Read the model definition and answer for the solid it produces. Units are mm, in the model's axes. A direction names the side the tool comes from. Coordinates: 2 decimals unless noted, no trailing zeros. Order: outer loops, then holes, each group sorted by start corner. A loop starts at its lowest first (then second) coordinate and runs counter-clockwise, first axis right, second up. Notation, with made-up numbers: M 2.5,-35.75 L 54.5,-35.75 A19 cw 54.5,-13.75 Z; hole C -34,49 d7. An arc over 180 degrees is marked long. Use a Markdown table: item, result. Add a question column.
1) Find section C-C on z = 15. Write down the section's boundary in (x, y).
2) The mould has two halves that part along X. Classify faces 1 (the face through (-9, 15, 19)), 2 (the face through (-20, 10, 0)), 3 (the face through (0, 10, -20)): released by +X, released by -X, zero draft, split by the parting line, or undercut.
3) Find section D-D on x = 5.5. Write down the section's boundary in (y, z), plus the area to 3 significant figures.
4) Find section A-A on x = -5. Write down the section's boundary in (y, z), plus the area to 3 significant figures.
5) Find section B-B on y = 7. Write down the section's boundary in (x, z), plus the area to 3 significant figures.
6) For faces 4 (the face through (-14.61, 8, 19)), 5 (the face through (0, 0, 0)), 6 (the face through (0, 11, -18)), determine the directions among +Z, -Z, +X, -X, +Y, -Y from which every point of the face is accessible in a straight line to the end or side of a thin tool.
7) Each of these flat-tipped pins is pushed along its axis until it touches: pin 1 Ø5.5 at (x, y) = (-8.5, 9.5) entering from +Z; pin 2 Ø11 at (x, z) = (-4, 4.5) entering from +Y. Where does it stop, or does it pass through?
8) Find the intervals of material crossed by probe 1 along Z at (x, y) = (9, 3.5); probe 2 along Y at (x, z) = (8, -2.5), in increasing order. Write a range as [from, to].
from build123d import *

# Parameters (mm, degrees)
SKETCH4_W           = 40
SKETCH4_H           = 40
BOSS_EXTRUDE3_DEPTH = 20
SHELL7_T            = -2
SKETCH5_W           = 12.32
SKETCH5_H           = 13
CUT_EXTRUDE1_DEPTH  = 2


with BuildPart() as part:
    # Sketch4 → Boss-Extrude3 (new body)
    with BuildSketch(Plane(origin=(0, 0, 0), x_dir=(1, 0, 0), z_dir=(0, 1, 0))):
        Rectangle(SKETCH4_W, SKETCH4_H)
    extrude(amount=BOSS_EXTRUDE3_DEPTH)

    # Shell7
    shell7_openings = [part.faces().sort_by_distance(p)[0] for p in [
        (0, 20, 0),
    ]]
    offset(amount=SHELL7_T, openings=shell7_openings, kind=Kind.INTERSECTION)

    # Sketch5 → Cut-Extrude1 (cut)
    with BuildSketch(Plane.XY.offset(20)):
        with Locations((-8.449687556, 8.5)):
            Rectangle(SKETCH5_W, SKETCH5_H)
    extrude(amount=-CUT_EXTRUDE1_DEPTH, mode=Mode.SUBTRACT)


solid = part.part
Check result:
| question | item | result |
|---|---|---|
| 1 | outline | M -20,0 L 20,0 L 20,20 L 18,20 L 18,2 L -18,2 L -18,20 L -20,20 Z |
| 2 | face 1 | undercut |
| 2 | face 2 | released by -X |
| 2 | face 3 | zero draft |
| 3 | outline | M 0,-20 L 20,-20 L 20,-18 L 2,-18 L 2,18 L 20,18 L 20,20 L 0,20 Z |
| 3 | area | 152 mm2 |
| 4 | outline | M 0,-20 L 20,-20 L 20,-18 L 2,-18 L 2,20 L 0,20 Z; M 15,18 L 20,18 L 20,20 L 15,20 Z |
| 4 | area | 126 mm2 |
| 5 | outline | M -20,-20 L 20,-20 L 20,20 L -2.29,20 L -2.29,18 L 18,18 L 18,-18 L -18,-18 L -18,18 L -14.61,18 L -14.61,20 L -20,20 Z |
| 5 | area | 279 mm2 |
| 6 | face 4 | +Z |
| 6 | face 5 | +Z, -Z, +X, -X, -Y |
| 6 | face 6 | +Y |
| 7 | pin 1 | stops at z = -18 |
| 7 | pin 2 | stops at y = 2 |
| 8 | probe 1 | z = [-20, -18], [18, 20] |
| 8 | probe 2 | y = [0, 2] |
